Could you check a few things on this drawing? It's one solid part, dimensions in mm from its lowest x, y, z. A direction names the side the tool comes from. Give positions to 0.01 mm unless a question says otherwise; leave off trailing zeros. Write each loop counter-clockwise with the first axis right and the second up, starting at its lowest first coordinate (ties: lowest second). Pieces come first, ordered by that corner, then holes. Notation, with made-up numbers: M 22,17 L 34,17 A28 cw 34,41 Z; hole C 59.5,-22.5 d4. An arc over 180 degrees is marked long. Answer as CSV lines item,"result". Start each with the question number.
Q1. Thinking about a two-plate mould opening in Z: for the marked faces 3, 4 and 5, which applies, +Z half, -Z half, draft (parallel to the pull), parting line (faces both ways), or undercut?
Q2. Suppose I cut it at D-D (x = 95). Write out the boundary of the cut face in (y, z).
Q3. Suppose I cut it at A-A (y = 16.25). Write out the boundary of the cut face in (x, z).
Q4. Suppose I cut it at B-B (y = 6). Write out the boundary of the cut face in (x, z), then the cut area to 3 significant figures.
Q5. For pin 1 (6 mm diameter, centred on y = 17, z = 34, fed in from -X); pin 2 (8 mm diameter, centred on y = 8.5, z = 9.5, fed in from +X); pin 3 (1 mm diameter, centred on x = 16.5, z = 16.5, fed in from -Y); pin 4 (5 mm diameter, centred on x = 63, y = 8.5, fed in from -Z), each with a flat end and sliding along its axis, tell me the tip position at first contact or that it passes through.
Q6. On a 3-axis mill with a long thin cutter (end or side, diameter ignored), from which of +Z, -Z, +X, -X, +Y, -Y can I reach the whole of each face in a straight line? I mean the marked faces 1 and 2. Say none if no direction works.
Q7. Suppose I cut it at C-C (x = 27.5). Write out the boundary of the cut face in (y, z).
Q8. If I drill on line 1 along X through (y, z) = (12, 25.5); line 2 along Z through (x, y) = (27.5, 11.5); line 3 along Z through (x, y) = (21.5, 16.5), over which ranges is the centre line in solid material (lowest first)?
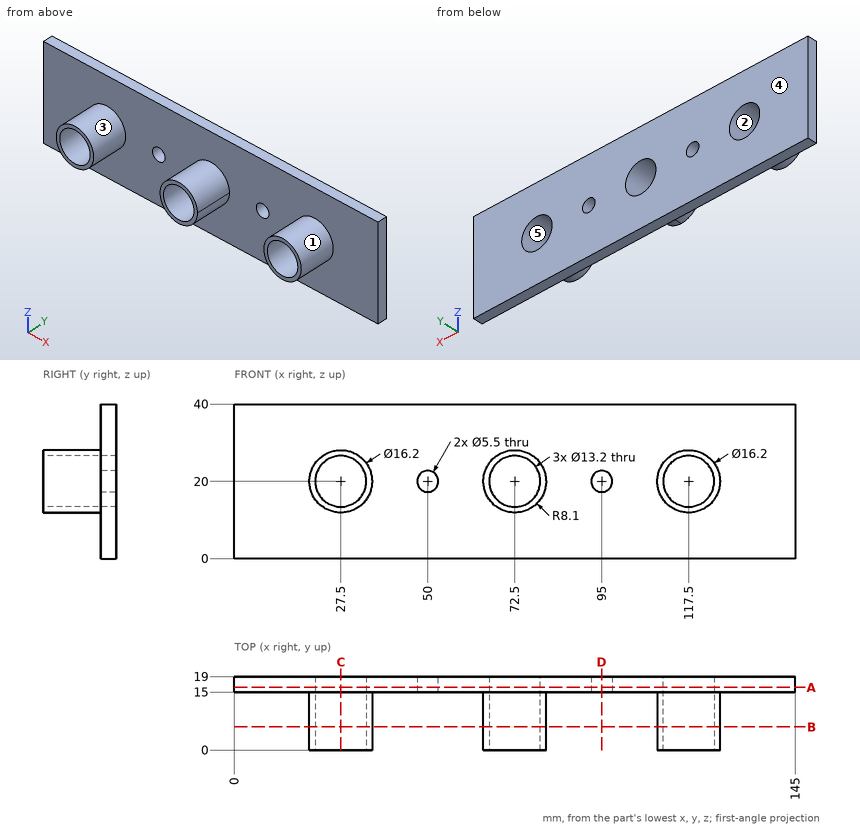
Resolved:
1,face 3,"parting line"
1,face 4,"draft"
1,face 5,"undercut"
2,outline,"M 15,0 L 19,0 L 19,17.25 L 15,17.25 Z; M 15,22.75 L 19,22.75 L 19,40 L 15,40 Z"
3,outline,"M 0,0 L 145,0 L 145,40 L 0,40 Z; hole C 27.5,20 d13.2; hole C 50,20 d5.5; hole C 72.5,20 d13.2; hole C 95,20 d5.5; hole C 117.5,20 d13.2"
4,outline,"C 27.5,20 d16.2; C 72.5,20 d16.2; C 117.5,20 d16.2; hole C 27.5,20 d13.2; hole C 72.5,20 d13.2; hole C 117.5,20 d13.2"
4,area,"208 mm^2"
5,pin 1,"x = 0"
5,pin 2,"x = 122.33"
5,pin 3,"y = 15"
5,pin 4,"z = 15.92"
6,face 1,"-Y"
6,face 2,"+Y, -Y"
7,outline,"M 0,11.9 L 15,11.9 L 15,0 L 19,0 L 19,13.4 L 0,13.4 Z; M 0,26.6 L 19,26.6 L 19,40 L 15,40 L 15,28.1 L 0,28.1 Z"
8,line 1,"21.55 to 23.85, 31.15 to 33.45, 66.55 to 68.85, 76.15 to 78.45, 111.55 to 113.85, 121.15 to 123.45"
8,line 2,"11.9 to 13.4, 26.6 to 28.1"
8,line 3,"0 to 17.25, 22.75 to 40"
